from build123d import *

# Parameters (mm, degrees)
F0_W     = 60
F0_H     = 23
F1_DEPTH = 25
F2_W     = 56
F2_H     = 46
F3_DEPTH = 22
F4_W     = 15
F4_H     = 2
F5_DEPTH = 4
F6_W     = 13
F6_H     = 3
F7_DEPTH = 2
F8_R     = 0.5


with BuildPart() as f1:
    # F0 (on Front) → F1 (new body, symmetric)
    with BuildSketch(Plane.XZ):
        Rectangle(F0_W, F0_H)
    extrude(amount=F1_DEPTH, both=True)

    # F2 (on face) → F3 (cut)
    with BuildSketch(Plane.XY.offset(11.5)):
        Rectangle(F2_W, F2_H)
    extrude(amount=-F3_DEPTH, mode=Mode.SUBTRACT)

    # F4 (on face) → F5 (join)
    with BuildSketch(Plane.XZ.offset(25)):
        Rectangle(F4_W, F4_H)
    extrude(amount=F5_DEPTH)

    # F6 (on face) → F7 (cut)
    with BuildSketch(Plane.XY.offset(1)):
        with Locations((0, -26.5)):
            Rectangle(F6_W, F6_H)
    extrude(amount=-F7_DEPTH, mode=Mode.SUBTRACT)

    # F8
    f8_edges = [f1.edges().sort_by_distance(p)[0] for p in [
        (-7.5, -29, 0),
        (7.5, -29, 0),
    ]]
    fillet(f8_edges, radius=F8_R)


solid = f1.part
Work out the finished part from the listing and answer in its coordinate system (mm). A direction names the side the tool comes from. Coordinates: 2 decimals unless noted, no trailing zeros. Loops run counter-clockwise (first coordinate to the right, second up) from the corner with the lowest first, then second, coordinate; pieces in that order, holes last. Notation, with made-up numbers: (-37.75, 88) -> (-27.75, 88) arc R14 cw to (-27.75, 99) -> close; hole circle Ø1 at (22.5, 84). An arc over 180 degrees is marked (long way). Answer as CSV lines item,"result".
1) The part is cut by section B-B (x = -2.5). Give the vertices of the cut face in (y, z).
A:
outline,"(-29, -1) -> (-28, -1) -> (-28, 1) -> (-29, 1) -> close; (-25, -11.5) -> (25, -11.5) -> (25, 11.5) -> (23, 11.5) -> (23, -10.5) -> (-23, -10.5) -> (-23, 11.5) -> (-25, 11.5) -> close"
2) Straight lines are drawn through the part: probe 1 along Y at (x, z) = (-5.5, 0.25); probe 2 along X at (y, z) = (12, -8.5); probe 3 along Y at (x, z) = (19, -6.25). For each, find the intervals that lie inside material, in ascending order.
A:
probe 1,"y = -29 to -28, -25 to -23, 23 to 25"
probe 2,"x = -30 to -28, 28 to 30"
probe 3,"y = -25 to -23, 23 to 25"
3) For a pull along X with two mould halves and no side action, classify faces 1 (the face through (7.5, -27, 0)), 2 (the face through (-6.5, -27, 0)), 3 (the face through (-0.1, -28.3, -1)), 4 (the face through (0, 0, -10.5)) as released by +X, released by -X, zero draft, split by the parting line, or undercut.
A:
face 1,"released by +X"
face 2,"undercut"
face 3,"zero draft"
face 4,"undercut"
4) The part is cut by section A-A (z = -3.25). Give the vertices of the cut face in (x, y).
A:
outline,"(-30, -25) -> (30, -25) -> (30, 25) -> (-30, 25) -> close; hole (-28, -23) -> (28, -23) -> (28, 23) -> (-28, 23) -> close"
5) The part is cut by section C-C (y = -8). Give the vertices of the cut face in (x, z).
A:
outline,"(-30, -11.5) -> (30, -11.5) -> (30, 11.5) -> (28, 11.5) -> (28, -10.5) -> (-28, -10.5) -> (-28, 11.5) -> (-30, 11.5) -> close"
6) Flat-ended cylindrical pins translate along their axes: pin 1 (1.6 mm diameter, centred on y = -27, z = 0.5, fed in from +X); pin 2 (1.6 mm diameter, centred on y = -26, z = -0.5, fed in from -X); pin 3 (1.2 mm diameter, centred on x = 0.5, y = -27.5, fed in from +Z). Find the tip coordinate at first contact, or state that the pin passes through.
A:
pin 1,"stops at x = 7.5"
pin 2,"stops at x = -7.5"
pin 3,"stops at z = 1"
7) For faces 5 (the face through (-0.1, -28.3, 1)), 6 (the face through (-28, 0, 1)), 7 (the face through (0, -29, 0)), 8 (the face through (-7.5, -27, 0)), 9 (the face through (6.5, -27, 0)), determine the directions among +Z, -Z, +X, -X, +Y, -Y from which every point of the face is accessible in a straight line to the end or side of a thin tool.
A:
face 5,"+Z, +X, -X, -Y"
face 6,"+Z"
face 7,"+Z, -Z, +X, -X, -Y"
face 8,"+Z, -Z, -X, -Y"
face 9,"+Z, -Z"
8) The part is cut by section D-D (x = -10). Give the vertices of the cut face in (y, z), and give its area (3 significant figures).
A:
outline,"(-25, -11.5) -> (25, -11.5) -> (25, 11.5) -> (23, 11.5) -> (23, -10.5) -> (-23, -10.5) -> (-23, 11.5) -> (-25, 11.5) -> close"
area,"138 mm²"
